Part model, mm, in its own coordinate system. A direction names the side the tool comes from. Give positions to 0.01 mm unless a question says otherwise; leave off trailing zeros. Order: outer loops, then holes, each group sorted by start corner. A loop starts at its lowest first (then second) coordinate and runs counter-clockwise, first axis right, second up.
1. Which spindle directions (+Z, -Z, +X, -X, +Y, -Y) get a long thin tool onto all of the face, cutting with end or side? Do faces 1 (the cylindrical face through (-10.88, 7.46, 6.16)), 2 (the cylindrical face through (15.9, 2.5, 10.6)), 3 (the cylindrical face through (0, 7, 11)). Say none if no direction does.
2. Slice it at B-B on y = 5.75. List the corners of the cut face in (x, z).
3. Slice it at D-D on x = -5.5. List the corners of the cut face in (y, z), and give its area (3 significant figures).
4. Mould opens along Z. For faces 4 (the cylindrical face through (-8.62, 7.46, -15.17)), 5 (the cylindrical face through (-17.45, 7.46, -0.12)), 6 (the flat face through (0, 5, -12)) say: +Z half, -Z half, draft (parallel to the pull), parting line (faces both ways), or undercut.
5. Probe line 1 (X direction, y = 4.25, z = 0); line 2 (X direction, y = 6.45, z = 7.5); line 3 (Y direction, x = -17, z = 18.5). List the from-to ranges inside material, lowest first.
6. Slice it at A-A on z = 0. List the corners of the cut face in (x, y).
7. Drop flat-ended pins along their axis: pin 1 Ø6.5 at (x, z) = (12.99, -7.5) entering from -Y; pin 2 Ø1.5 at (y, z) = (3.5, 6) entering from -X; pin 3 Ø6 at (y, z) = (5, -10.5) entering from +X. Give the stop position or say it passes through.
8. Slice it at C-C on z = -18.5. List the corners of the cut face in (x, y).
from build123d import *

# Parameters (mm, degrees)
SKETCH1_R           = 27
BOSS_EXTRUDE1_DEPTH = 5
SKETCH2_R           = 17.45
BOSS_EXTRUDE2_DEPTH = 5
SKETCH3_R           = 2.5
CUT_EXTRUDE1_DEPTH  = 15
SKETCH5_R           = 11
CUT_EXTRUDE2_DEPTH  = 6.5
SKETCH6_R           = 1.689113582
CUT_EXTRUDE3_DEPTH  = 36.5
SKETCH7_R           = 5
CUT_EXTRUDE4_DEPTH  = 36.5
SKETCH8_R           = 4.25
CUT_EXTRUDE5_DEPTH  = 5
CUT_EXTRUDE6_REACH  = 40.733
SKETCH10_R          = 7.574183751


with BuildPart() as part:
    # Sketch1 → Boss-Extrude1 (new body)
    with BuildSketch(Plane(origin=(0, 0, 0), x_dir=(1, 0, 0), z_dir=(0, 1, 0))):
        with Locations(Location((0, 0, 0), (0, 0, 270))):
            Circle(SKETCH1_R)
    extrude(amount=BOSS_EXTRUDE1_DEPTH)

    # Sketch2 → Boss-Extrude2 (add)
    with BuildSketch(Plane(origin=(0, 5, 0), x_dir=(1, 0, 0), z_dir=(0, 1, 0))):
        with Locations(Location((0, 0, 0), (0, 0, 270))):
            Circle(SKETCH2_R)
    extrude(amount=BOSS_EXTRUDE2_DEPTH)

    # Sketch3 → Cut-Extrude1 (cut)
    with BuildSketch(Plane.XZ):
        with Locations(Location((0, 15, 0), (0, 0, 270))):
            Circle(SKETCH3_R)
        with Locations(Location((12.990381057, 7.5, 0), (0, 0, 270))):
            Circle(SKETCH3_R)
        with Locations(Location((12.990381057, -7.5, 0), (0, 0, 270))):
            Circle(SKETCH3_R)
        with Locations(Location((0, -15, 0), (0, 0, 270))):
            Circle(SKETCH3_R)
        with Locations(Location((-12.990381057, -7.5, 0), (0, 0, 270))):
            Circle(SKETCH3_R)
        with Locations(Location((-12.990381057, 7.5, 0), (0, 0, 270))):
            Circle(SKETCH3_R)
    extrude(amount=-CUT_EXTRUDE1_DEPTH, mode=Mode.SUBTRACT)

    # Sketch5 → Cut-Extrude2 (cut)
    with BuildSketch(Plane(origin=(0, 10, 0), x_dir=(1, 0, 0), z_dir=(0, 1, 0))):
        with Locations(Location((0, 0, 0), (0, 0, 270))):
            Circle(SKETCH5_R)
    extrude(amount=-CUT_EXTRUDE2_DEPTH, mode=Mode.SUBTRACT)

    # Sketch6 → Cut-Extrude3 (cut)
    with BuildSketch(Plane(origin=(0, 10, 0), x_dir=(1, 0, 0), z_dir=(0, 1, 0))):
        with Locations(Location((-11, 0, 0), (0, 0, 270))):
            Circle(SKETCH6_R)
        with Locations(Location((-5.5, 9.526279442, 0), (0, 0, 270))):
            Circle(SKETCH6_R)
        with Locations(Location((5.5, 9.526279442, 0), (0, 0, 270))):
            Circle(SKETCH6_R)
        with Locations(Location((11, 0, 0), (0, 0, 270))):
            Circle(SKETCH6_R)
        with Locations(Location((5.5, -9.526279442, 0), (0, 0, 270))):
            Circle(SKETCH6_R)
        with Locations(Location((-5.5, -9.526279442, 0), (0, 0, 270))):
            Circle(SKETCH6_R)
    extrude(amount=-CUT_EXTRUDE3_DEPTH, mode=Mode.SUBTRACT)

    # Sketch7 → Cut-Extrude4 (cut)
    with BuildSketch(Plane(origin=(0, 3.5, 0), x_dir=(1, 0, 0), z_dir=(0, 1, 0))):
        with Locations(Location((0, 0, 0), (0, 0, 270))):
            Circle(SKETCH7_R)
    extrude(amount=-CUT_EXTRUDE4_DEPTH, mode=Mode.SUBTRACT)

    # Sketch8 → Cut-Extrude5 (cut)
    with BuildSketch(Plane.XZ):
        with Locations(Location((0, 15, 0), (0, 0, 270))):
            Circle(SKETCH8_R)
        with Locations(Location((12.990381057, 7.5, 0), (0, 0, 270))):
            Circle(SKETCH8_R)
        with Locations(Location((12.990381057, -7.5, 0), (0, 0, 270))):
            Circle(SKETCH8_R)
        with Locations(Location((0, -15, 0), (0, 0, 270))):
            Circle(SKETCH8_R)
        with Locations(Location((-12.990381057, -7.5, 0), (0, 0, 270))):
            Circle(SKETCH8_R)
        with Locations(Location((-12.990381057, 7.5, 0), (0, 0, 270))):
            Circle(SKETCH8_R)
    extrude(amount=-CUT_EXTRUDE5_DEPTH, mode=Mode.SUBTRACT)

    # Sketch10 → Cut-Extrude6 (cut, up to next)
    with BuildSketch(Plane(origin=(0, 3.5, 0), x_dir=(1, 0, 0), z_dir=(0, 1, 0)), mode=Mode.PRIVATE) as cut_extrude6_sk1:
        with Locations(Location((0, 0, 0), (0, 0, 270))):
            Circle(SKETCH10_R)
    cut_extrude6_tool1 = extrude(cut_extrude6_sk1.sketch, amount=-CUT_EXTRUDE6_REACH, mode=Mode.PRIVATE) & part.part
    add(cut_extrude6_tool1.solids().sort_by_distance((0, 3.5, 0))[0], mode=Mode.SUBTRACT)


solid = part.part
Data:
1. face 1: +Y, -Y
1. face 2: -Y
1. face 3: +Y
2. outline: (-15.37, -8.26) arc R2.5 cw (long way) to (-14.84, -9.19) arc R17.45 ccw to (-0.54, -17.44) arc R2.5 cw (long way) to (0.54, -17.44) arc R17.45 ccw to (14.84, -9.19) arc R2.5 cw (long way) to (15.37, -8.26) arc R17.45 ccw to (15.37, 8.26) arc R2.5 cw (long way) to (14.84, 9.19) arc R17.45 ccw to (0.54, 17.44) arc R2.5 cw (long way) to (-0.54, 17.44) arc R17.45 ccw to (-14.84, 9.19) arc R2.5 cw (long way) to (-15.37, 8.26) arc R17.45 ccw to start; hole (-10.87, -1.68) arc R11 ccw to (-6.89, -8.57) arc R1.69 ccw (long way) to (-3.98, -10.26) arc R11 ccw to (3.98, -10.26) arc R1.69 ccw (long way) to (6.89, -8.57) arc R11 ccw to (10.87, -1.68) arc R1.69 ccw (long way) to (10.87, 1.68) arc R11 ccw to (6.89, 8.57) arc R1.69 ccw (long way) to (3.98, 10.26) arc R11 ccw to (-3.98, 10.26) arc R1.69 ccw (long way) to (-6.89, 8.57) arc R11 ccw to (-10.87, 1.68) arc R1.69 ccw (long way) to start
3. outline: (0, -26.43) - (5, -26.43) - (5, -16.56) - (10, -16.56) - (10, -11.22) - (0, -11.22) - close; (0, -7.84) - (3.5, -7.84) - (3.5, -5.21) - (0, -5.21) - close; (0, 5.21) - (3.5, 5.21) - (3.5, 7.84) - (0, 7.84) - close; (0, 11.22) - (10, 11.22) - (10, 16.56) - (5, 16.56) - (5, 26.43) - (0, 26.43) - close
3. area: 224 mm2
4. face 4: -Z half
4. face 5: parting line
4. face 6: undercut
5. line 1: x = -27 to -12.69, 12.69 to 27
5. line 2: x = -15.76 to -15.49, -10.49 to -8.05, 8.05 to 10.49, 15.49 to 15.76
5. line 3: y = 0 to 5
6. outline: (-27, 0) - (-12.69, 0) - (-12.69, 10) - (-17.45, 10) - (-17.45, 5) - (-27, 5) - close; (-9.31, 0) - (-7.57, 0) - (-7.57, 3.5) - (-9.31, 3.5) - close; (7.57, 0) - (9.31, 0) - (9.31, 3.5) - (7.57, 3.5) - close; (12.69, 0) - (27, 0) - (27, 5) - (17.45, 5) - (17.45, 10) - (12.69, 10) - close
7. pin 1: stops at y = 5
7. pin 2: stops at x = -26.48
7. pin 3: stops at x = 25.94
8. outline: (-19.67, 0) - (-2.41, 0) - (-2.41, 5) - (-19.67, 5) - close; (2.41, 0) - (19.67, 0) - (19.67, 5) - (2.41, 5) - close
